from build123d import *

# Parameters (mm, degrees)
IZIM2_W                     = 60
IZIM2_H                     = 40
Y_KSEKLIK_EKSTR_ZYON1_DEPTH = 60
BO_ALTMA1_T                 = -2
KES_EKSTR_ZYON2_REACH       = 95.808
IZIM4_R                     = 2
IZIM4_W                     = 40
IZIM4_H                     = 20
KES_EKSTR_ZYON3_REACH       = 95.808
IZIM5_R                     = 2
KES_EKSTR_ZYON4_REACH       = 95.808
IZIM6_R                     = 4


with BuildPart() as part:
    # Çizim2 → Yükseklik-Ekstrüzyon1 (new body)
    with BuildSketch(Plane.XY):
        with Locations((30, 20)):
            Rectangle(IZIM2_W, IZIM2_H)
    extrude(amount=Y_KSEKLIK_EKSTR_ZYON1_DEPTH)

    # İç Boşaltma1
    bo_altma1_openings = [part.faces().sort_by_distance(p)[0] for p in [
        (30, 40, 30),
    ]]
    offset(amount=BO_ALTMA1_T, openings=bo_altma1_openings, kind=Kind.INTERSECTION)

    # Çizim4 → Kes-Ekstrüzyon2 (cut, up to next)
    with BuildSketch(Plane(origin=(0, 0, 0), x_dir=(-1, 0, 0), z_dir=(0, 0, -1)), mode=Mode.PRIVATE) as kes_ekstr_zyon2_sk1:
        with Locations((-53.5, 25)):
            Circle(IZIM4_R)
    kes_ekstr_zyon2_tool1 = extrude(kes_ekstr_zyon2_sk1.sketch, amount=-KES_EKSTR_ZYON2_REACH, mode=Mode.PRIVATE) & part.part
    # Çizim4 → Kes-Ekstrüzyon2 (cut, up to next)
    with BuildSketch(Plane(origin=(0, 0, 0), x_dir=(-1, 0, 0), z_dir=(0, 0, -1)), mode=Mode.PRIVATE) as kes_ekstr_zyon2_sk2:
        with Locations((-53.5, 15)):
            Circle(IZIM4_R)
    kes_ekstr_zyon2_tool2 = extrude(kes_ekstr_zyon2_sk2.sketch, amount=-KES_EKSTR_ZYON2_REACH, mode=Mode.PRIVATE) & part.part
    # Çizim4 → Kes-Ekstrüzyon2 (cut, up to next)
    with BuildSketch(Plane(origin=(0, 0, 0), x_dir=(-1, 0, 0), z_dir=(0, 0, -1)), mode=Mode.PRIVATE) as kes_ekstr_zyon2_sk3:
        with Locations((-6.5, 15)):
            Circle(IZIM4_R)
    kes_ekstr_zyon2_tool3 = extrude(kes_ekstr_zyon2_sk3.sketch, amount=-KES_EKSTR_ZYON2_REACH, mode=Mode.PRIVATE) & part.part
    # Çizim4 → Kes-Ekstrüzyon2 (cut, up to next)
    with BuildSketch(Plane(origin=(0, 0, 0), x_dir=(-1, 0, 0), z_dir=(0, 0, -1)), mode=Mode.PRIVATE) as kes_ekstr_zyon2_sk4:
        with Locations((-6.5, 25)):
            Circle(IZIM4_R)
    kes_ekstr_zyon2_tool4 = extrude(kes_ekstr_zyon2_sk4.sketch, amount=-KES_EKSTR_ZYON2_REACH, mode=Mode.PRIVATE) & part.part
    # Çizim4 → Kes-Ekstrüzyon2 (cut, up to next)
    with BuildSketch(Plane(origin=(0, 0, 0), x_dir=(-1, 0, 0), z_dir=(0, 0, -1)), mode=Mode.PRIVATE) as kes_ekstr_zyon2_sk5:
        with Locations((-30, 20)):
            Rectangle(IZIM4_W, IZIM4_H)
    kes_ekstr_zyon2_tool5 = extrude(kes_ekstr_zyon2_sk5.sketch, amount=-KES_EKSTR_ZYON2_REACH, mode=Mode.PRIVATE) & part.part
    add(kes_ekstr_zyon2_tool1.solids().sort_by_distance((53.5, 25, 0))[0], mode=Mode.SUBTRACT)
    add(kes_ekstr_zyon2_tool2.solids().sort_by_distance((53.5, 15, 0))[0], mode=Mode.SUBTRACT)
    add(kes_ekstr_zyon2_tool3.solids().sort_by_distance((6.5, 15, 0))[0], mode=Mode.SUBTRACT)
    add(kes_ekstr_zyon2_tool4.solids().sort_by_distance((6.5, 25, 0))[0], mode=Mode.SUBTRACT)
    add(kes_ekstr_zyon2_tool5.solids().sort_by_distance((30, 20, 0))[0], mode=Mode.SUBTRACT)

    # Çizim5 → Kes-Ekstrüzyon3 (cut, up to next)
    with BuildSketch(Plane.XZ, mode=Mode.PRIVATE) as kes_ekstr_zyon3_sk1:
        with Locations(Location((30, 30, 0), (0, 0, 270))):
            Circle(IZIM5_R)
    kes_ekstr_zyon3_tool1 = extrude(kes_ekstr_zyon3_sk1.sketch, amount=-KES_EKSTR_ZYON3_REACH, mode=Mode.PRIVATE) & part.part
    # Çizim5 → Kes-Ekstrüzyon3 (cut, up to next)
    with BuildSketch(Plane.XZ, mode=Mode.PRIVATE) as kes_ekstr_zyon3_sk2:
        with Locations(Location((38, 30, 0), (0, 0, 270))):
            Circle(IZIM5_R)
    kes_ekstr_zyon3_tool2 = extrude(kes_ekstr_zyon3_sk2.sketch, amount=-KES_EKSTR_ZYON3_REACH, mode=Mode.PRIVATE) & part.part
    # Çizim5 → Kes-Ekstrüzyon3 (cut, up to next)
    with BuildSketch(Plane.XZ, mode=Mode.PRIVATE) as kes_ekstr_zyon3_sk3:
        with Locations(Location((30, 38, 0), (0, 0, 270))):
            Circle(IZIM5_R)
    kes_ekstr_zyon3_tool3 = extrude(kes_ekstr_zyon3_sk3.sketch, amount=-KES_EKSTR_ZYON3_REACH, mode=Mode.PRIVATE) & part.part
    # Çizim5 → Kes-Ekstrüzyon3 (cut, up to next)
    with BuildSketch(Plane.XZ, mode=Mode.PRIVATE) as kes_ekstr_zyon3_sk4:
        with Locations(Location((30, 22, 0), (0, 0, 90))):
            Circle(IZIM5_R)
    kes_ekstr_zyon3_tool4 = extrude(kes_ekstr_zyon3_sk4.sketch, amount=-KES_EKSTR_ZYON3_REACH, mode=Mode.PRIVATE) & part.part
    # Çizim5 → Kes-Ekstrüzyon3 (cut, up to next)
    with BuildSketch(Plane.XZ, mode=Mode.PRIVATE) as kes_ekstr_zyon3_sk5:
        with Locations(Location((22, 30, 0), (0, 0, 90))):
            Circle(IZIM5_R)
    kes_ekstr_zyon3_tool5 = extrude(kes_ekstr_zyon3_sk5.sketch, amount=-KES_EKSTR_ZYON3_REACH, mode=Mode.PRIVATE) & part.part
    add(kes_ekstr_zyon3_tool1.solids().sort_by_distance((30, 0, 30))[0], mode=Mode.SUBTRACT)
    add(kes_ekstr_zyon3_tool2.solids().sort_by_distance((38, 0, 30))[0], mode=Mode.SUBTRACT)
    add(kes_ekstr_zyon3_tool3.solids().sort_by_distance((30, 0, 38))[0], mode=Mode.SUBTRACT)
    add(kes_ekstr_zyon3_tool4.solids().sort_by_distance((30, 0, 22))[0], mode=Mode.SUBTRACT)
    add(kes_ekstr_zyon3_tool5.solids().sort_by_distance((22, 0, 30))[0], mode=Mode.SUBTRACT)

    # Çizim6 → Kes-Ekstrüzyon4 (cut, up to next)
    with BuildSketch(Plane.XY.offset(60), mode=Mode.PRIVATE) as kes_ekstr_zyon4_sk1:
        with Locations((20, 20)):
            Circle(IZIM6_R)
    kes_ekstr_zyon4_tool1 = extrude(kes_ekstr_zyon4_sk1.sketch, amount=-KES_EKSTR_ZYON4_REACH, mode=Mode.PRIVATE) & part.part
    # Çizim6 → Kes-Ekstrüzyon4 (cut, up to next)
    with BuildSketch(Plane.XY.offset(60), mode=Mode.PRIVATE) as kes_ekstr_zyon4_sk2:
        with Locations(Location((40, 20, 0), (0, 0, 180))):
            Circle(IZIM6_R)
    kes_ekstr_zyon4_tool2 = extrude(kes_ekstr_zyon4_sk2.sketch, amount=-KES_EKSTR_ZYON4_REACH, mode=Mode.PRIVATE) & part.part
    add(kes_ekstr_zyon4_tool1.solids().sort_by_distance((20, 20, 60))[0], mode=Mode.SUBTRACT)
    add(kes_ekstr_zyon4_tool2.solids().sort_by_distance((40, 20, 60))[0], mode=Mode.SUBTRACT)


solid = part.part
Part model, mm, in its own coordinate system. A direction names the side the tool comes from. Round coordinates to 2 decimals unless told otherwise and drop trailing zeros. Write each loop counter-clockwise with the first axis right and the second up, starting at its lowest first coordinate (ties: lowest second). Pieces come first, ordered by that corner, then holes. Notation, with made-up numbers: (46, 87.5) - (89, 87.5) arc R29 ccw to (89, 117.5) - close; hole circle Ø8 at (-32.75, 0.5). An arc over 180 degrees is marked (long way). Use CSV: the item, a comma, the result in double quotes.
Item 1: Flat gauge pins, fed straight in: P1, Ø5, axis at x = 43, y = 14, coming from the -Z side; P2, Ø2.5, axis at x = 30, z = 38, coming from the -Y side. Where does each tip first touch, or does it go through?
Results list:
P1,"stops at z = 58"
P2,"passes through"
Item 2: Slice it at D-D, the plane x = 17. Write the cut outline in (y, z).
Results list:
outline,"(0, 0) - (10, 0) - (10, 2) - (2, 2) - (2, 58) - (17.35, 58) - (17.35, 60) - (0, 60) - close; (22.65, 58) - (40, 58) - (40, 60) - (22.65, 60) - close; (30, 0) - (40, 0) - (40, 2) - (30, 2) - close"
Item 3: Slice it at A-A, the plane x = 30. Write the cut outline in (y, z), then the cut area to 3 significant figures.
Results list:
outline,"(0, 0) - (10, 0) - (10, 2) - (2, 2) - (2, 20) - (0, 20) - close; (0, 24) - (2, 24) - (2, 28) - (0, 28) - close; (0, 32) - (2, 32) - (2, 36) - (0, 36) - close; (0, 40) - (2, 40) - (2, 58) - (40, 58) - (40, 60) - (0, 60) - close; (30, 0) - (40, 0) - (40, 2) - (30, 2) - close"
area,"208 mm²"
Item 4: Wall check: L1, parallel to X at y = 1.3, z = 30; L2, parallel to X at y = 5, z = 27.5. Give the ranges that are in metal, low to high.
Results list:
L1,"x = 0 to 20, 24 to 28, 32 to 36, 40 to 60"
L2,"x = 0 to 2, 58 to 60"
Item 5: Tool access for faces 1 (the flat face through (30, 9, 2)), 2 (the cylindrical face through (36.226, 0.986, 29.077)), 3 (the cylindrical face through (6.76, 16.983, 0.986)): list every direction of +Z, -Z, +X, -X, +Y, -Y with a clear straight run to the whole face (end or side of a thin tool).
Results list:
face 1,"+Y"
face 2,"+Y, -Y"
face 3,"-Z"
Item 6: Slice it at C-C, the plane z = 22. Write the cut outline in (x, y), then the cut area to 3 significant figures.
Results list:
outline,"(0, 0) - (28, 0) - (28, 2) - (2, 2) - (2, 40) - (0, 40) - close; (32, 0) - (60, 0) - (60, 40) - (58, 40) - (58, 2) - (32, 2) - close"
area,"264 mm²"
Item 7: Slice it at B-B, the plane y = 26. Write the cut outline in (x, z), then the cut area to 3 significant figures.
Results list:
outline,"(0, 0) - (4.77, 0) - (4.77, 2) - (2, 2) - (2, 58) - (58, 58) - (58, 2) - (55.23, 2) - (55.23, 0) - (60, 0) - (60, 60) - (0, 60) - close; (8.23, 0) - (10, 0) - (10, 2) - (8.23, 2) - close; (50, 0) - (51.77, 0) - (51.77, 2) - (50, 2) - close"
area,"370 mm²"
Item 8: Pull direction Z, two halves, no side cores. Call faces 4 (the flat face through (60, 20, 30)), 5 (the cylindrical face through (32, 1, 22)), 6 (the flat face through (30, 20, 60)): pulls with the +Z half, pulls with the -Z half, needs draft (parallel to the pull), parting line crosses it, or undercut.
Results list:
face 4,"needs draft"
face 5,"undercut"
face 6,"pulls with the +Z half"
